The listing builds one solid part. Answer for the finished solid, in the listing's coordinates (mm). A direction names the side the tool comes from. Coordinates: 2 decimals unless noted, no trailing zeros. Order: outer loops, then holes, each group sorted by start corner. A loop starts at its lowest first (then second) coordinate and runs counter-clockwise, first axis right, second up. Notation, with made-up numbers: (-37, 75) -> (2, 75) arc R11 cw to (2, 82) -> close; hole circle Ø8 at (-10.75, 50). An arc over 180 degrees is marked (long way). Return JSON: item names as keys, results as strings.
Autodesk Inventor part; units mm, degrees
ref_plane "YZ Plane" through (0, 0, 0) normal (1, 0, 0) x (0, 1, 0)
ref_plane "XZ Plane" through (0, 0, 0) normal (0, 1, 0) x (-1, 0, 0)
ref_plane "XY Plane" through (0, 0, 0) normal (0, 0, 1) x (1, 0, 0)
sketch "Эскиз1" plane through (0, 0, 0) normal (0, 0, 1) x (1, 0, 0)
  line L0 (-26.85, 17.75) -> (26.85, 17.75)
  line L1 (26.85, 17.75) -> (26.85, -17.75)
  line L2 (26.85, -17.75) -> (-26.85, -17.75)
  line L3 (-26.85, -17.75) -> (-26.85, 17.75)
  line L4 (-26.85, 17.75) -> (26.85, -17.75) construction
  line L5 (26.85, 17.75) -> (-26.85, -17.75) construction
  point P0 (0, 0)
  dimension "d0" = 53.7
  dimension "d1" = 35.5
extrude "Выдавливание1" add sketch "Эскиз1" along normal blind 3.2
sketch "Эскиз2" plane through (0, 0, 0) normal (0, 0, -1) x (-1, 0, 0)
  line L0 (31.65, -16.5) -> (26.85, -16.5)
  line L1 (26.85, -16.5) -> (26.85, 16.5)
  line L2 (26.85, 16.5) -> (31.65, 16.5)
  line L3 (31.65, 16.5) -> (31.65, -16.5)
  line L4 (31.65, -16.5) -> (26.85, 16.5) construction
  line L5 (26.85, -16.5) -> (31.65, 16.5) construction
  line L6 (26.85, 17.75) -> (26.85, -17.75)
  point P0 (0, 0)
  point P1 (29.25, 0)
  point P2 (26.85, 0)
  dimension "d4" = 4.8
  dimension "d5" = 33
extrude "Выдавливание2" add sketch "Эскиз2" against normal blind 18.5
sketch "Эскиз3" plane through (0, 0, 3.2) normal (0, 0, 1) x (1, 0, 0)
  line L0 (-1.65, 20) -> (26.85, 20)
  line L1 (26.85, 20) -> (26.85, -20)
  line L2 (26.85, -20) -> (-1.65, -20)
  line L3 (-1.65, -20) -> (-1.65, 20)
  line L4 (-1.65, 20) -> (26.85, -20) construction
  line L5 (26.85, 20) -> (-1.65, -20) construction
  line L6 (26.85, -17.75) -> (26.85, 17.75)
  line L7 (-24.15, 20) -> (-7.15, 20)
  line L8 (-7.15, 20) -> (-7.15, -20)
  line L9 (-7.15, -20) -> (-24.15, -20)
  line L10 (-24.15, -20) -> (-24.15, 20)
  line L11 (-24.15, 20) -> (-7.15, -20) construction
  line L12 (-7.15, 20) -> (-24.15, -20) construction
  point P0 (0, 0)
  point P1 (12.6, 0)
  point P2 (26.85, 0)
  point P3 (-15.65, 0)
  dimension "d8" = 28.5
  dimension "d9" = 40
  dimension "d10" = 17
  dimension "d11" = 40
  dimension "d12" = 5.5
extrude "Выдавливание3" add sketch "Эскиз3" against normal blind 1.2
sketch "Эскиз4" plane through (0, 0, 0) normal (0, 0, -1) x (-1, 0, 0)
  circle A0 centre (-9.85, 0) radius 12
  line L0 (-26.85, -17.75) -> (-26.85, 17.75)
  circle A1 centre (-24.85, 3) radius 2
  circle A2 centre (-24.85, 3) radius 1.2
  line L1 (-9.85, 0) -> (-9.85, 16.0932) construction
  circle A3 centre (5.15, 3) radius 2
  circle A4 centre (5.15, 3) radius 1.2
  line L2 (1.65, 20) -> (-26.85, 20)
  point P0 (0, 0)
  dimension "d15" = 24
  dimension "d16" = 17
  dimension "d17" = 4
  dimension "d18" = 2.4
  dimension "d19" = 30
  dimension "d20" = 17
extrude "Выдавливание4" cut sketch "Эскиз4" against normal up to next contours A0
extrude "Выдавливание5" add sketch "Эскиз4" along normal blind 1.8 contours A1 | A3
extrude "Выдавливание6" cut sketch "Эскиз4" against normal up to next contours A2 | A4
sketch "Эскиз5" plane through (-31.65, -16.5, 0) normal (-1, 0, 0) x (0, 0, 1)
  circle A0 centre (10.968, 7.5) radius 4.5
  line L0 (0, 0) -> (18.5, 0)
  point P0 (0, 16.5)
  dimension "d27" = 9
  dimension "d28" = 7.5
extrude "Выдавливание7" cut sketch "Эскиз5" against normal up to next
fillet "Сопряжение1" radius 2 10 edges at (-29.25, -16.5, 18.5) (-29.25, 16.5, 18.5) (-31.65, -16.5, 9.25) (-31.65, 16.5, 9.25) (26.85, 20, 2.6) (26.85, 17.75, 1) (26.85, -17.75, 1) (26.85, -20, 2.6) (-26.85, 17.75, 1.6) (-26.85, -17.75, 1.6)
properties part number "ЛЦМК000002.00.00.00.00.15"
1. The part is cut by section A-A on x = -5.15. Give the vertices of the cut face in (y, z), and give its area (3 significant figures).
Answer block:
{"outline": "(-17.75, 0) -> (1, 0) -> (1, -1.8) -> (1.8, -1.8) -> (1.8, 3.2) -> (-17.75, 3.2) -> close; (4.2, -1.8) -> (5, -1.8) -> (5, 0) -> (17.75, 0) -> (17.75, 3.2) -> (4.2, 3.2) -> close", "area": "109 mm2"}
2. Consider line 1 (Y direction, x = 24.85, z = 0.5); line 2 (Z direction, x = -21, y = -7); line 3 (X direction, y = -4, z = 17.75). Determine where each line is inside the solid, lowest interval first. Write a range as from..to.
Answer block:
{"line 1": "y = -17.75..1.8, 4.2..17.75", "line 2": "z = 0..3.2", "line 3": "x = -31.65..-26.85"}
3. The part is cut by section C-C on z = 8.5. Give the vertices of the cut face in (x, y).
Answer block:
{"outline": "(-31.65, -14.5) arc R2 ccw to (-29.65, -16.5) -> (-26.85, -16.5) -> (-26.85, -12.76) -> (-31.65, -12.76) -> close; (-31.65, -5.24) -> (-26.85, -5.24) -> (-26.85, 16.5) -> (-29.65, 16.5) arc R2 ccw to (-31.65, 14.5) -> close"}
4. Each of these flat-tipped pins is pushed along its axis until it touches: pin 1 Ø5 at (y, z) = (-12, 13.5) entering from +X; pin 2 Ø3 at (x, z) = (-28.5, 10) entering from -Y; pin 3 Ø1.5 at (x, y) = (18, 6.5) entering from -Z; pin 4 Ø20 at (x, y) = (-12, 1) entering from +Z. Where does it stop, or does it pass through?
Answer block:
{"pin 1": "stops at x = -26.85", "pin 2": "stops at y = -16.5", "pin 3": "passes through", "pin 4": "stops at z = 3.2"}
5. Determine the mould class of faces 6 (the face through (-29.28, -7.65, 15.26)), 7 (the face through (12, -20, 3)), 8 (the face through (-1.596, 3.604, 1.578)), 9 (the face through (-1.65, -19, 3)) for opening direction Y: pulls with the +Y half, pulls with the -Y half, needs draft (parallel to the pull), parting line crosses it, or undercut.
Answer block:
{"face 6": "undercut", "face 7": "pulls with the -Y half", "face 8": "undercut", "face 9": "needs draft"}
6. The part is cut by section D-D on x = -20. Give the vertices of the cut face in (y, z), and give its area (3 significant figures).
Answer block:
{"outline": "(-20, 2) -> (-17.75, 2) -> (-17.75, 0) -> (17.75, 0) -> (17.75, 2) -> (20, 2) -> (20, 3.2) -> (-20, 3.2) -> close", "area": "119 mm2"}
7. The part is cut by section B-B on y = 0. Give the vertices of the cut face in (x, z).
Answer block:
{"outline": "(-31.65, 0) -> (-2.15, 0) -> (-2.15, 3.2) -> (-26.85, 3.2) -> (-26.85, 18.5) -> (-31.65, 18.5) -> close; (21.85, 0) -> (26.85, 0) -> (26.85, 3.2) -> (21.85, 3.2) -> close"}
8. For faces 1 (the face through (-6, 0, 3.2)), 2 (the face through (22.942, 2.399, -0.887)), 3 (the face through (-7.15, -19, 3)), 4 (the face through (26.28, -17.15, 0.99)), 5 (the face through (-24.15, -19, 3)), determine the directions among +Z, -Z, +X, -X, +Y, -Y from which every point of the face is accessible in a straight line to the end or side of a thin tool.
Answer block:
{"face 1": "+Z, +X, +Y, -Y", "face 2": "-Z", "face 3": "+Z, -Z, -Y", "face 4": "-Z, +X, -Y", "face 5": "+Z, -Z, -X, -Y"}
